The figure shows three views and two pictorial views of one solid part (mm, origin at its lowest corner). Answer the questions. Coordinates: 2 decimals unless noted, no trailing zeros. Order: outer loops, then holes, each group sorted by start corner. A loop starts at its lowest first (then second) coordinate and runs counter-clockwise, first axis right, second up. Notation, with made-up numbers: (73.25, -9.5) - (96.25, -9.5) arc R18 ccw to (96.25, 19.5) - close; hole circle Ø7 at (-17.5, 43.25). An arc over 180 degrees is marked (long way). Use one line per item in the form item = value. Start each with the question number.
Item 1: Section D-D, the plane y = 0.6 is taken. Count the separate pieces of the cut face and the enclosed holes in it, and give its area (3 significant figures).
Item 2: Section A-A, the plane z = 70 is taken. Write down the section's boundary in (x, y).
Item 3: Each of these flat-tipped pins is pushed along its axis until it touches: pin 1 Ø1.5 at (y, z) = (1, 108) entering from +X (1 decimal); pin 2 Ø5.5 at (x, z) = (11, 70) entering from +Y; pin 3 Ø2 at (y, z) = (2.5, 91.5) entering from +X; pin 4 Ø1.5 at (y, z) = (1.5, 37) entering from -X. Where does it stop, or does it pass through?
Item 4: Section B-B, the plane z = 11 is taken. Write down the section's boundary in (x, y), and give its area (3 significant figures).
Item 5: Consider line 1 along X through (y, z) = (1.85, 70); line 2 along Z through (x, y) = (109, 2.3); line 3 along Z through (x, y) = (28, 1.7). Determine where each line is inside the solid, lowest interval first. Write a range as [from, to].
Item 6: Section C-C, the plane x = 129 is taken. Write down the section's boundary in (y, z), and give its area (3 significant figures).
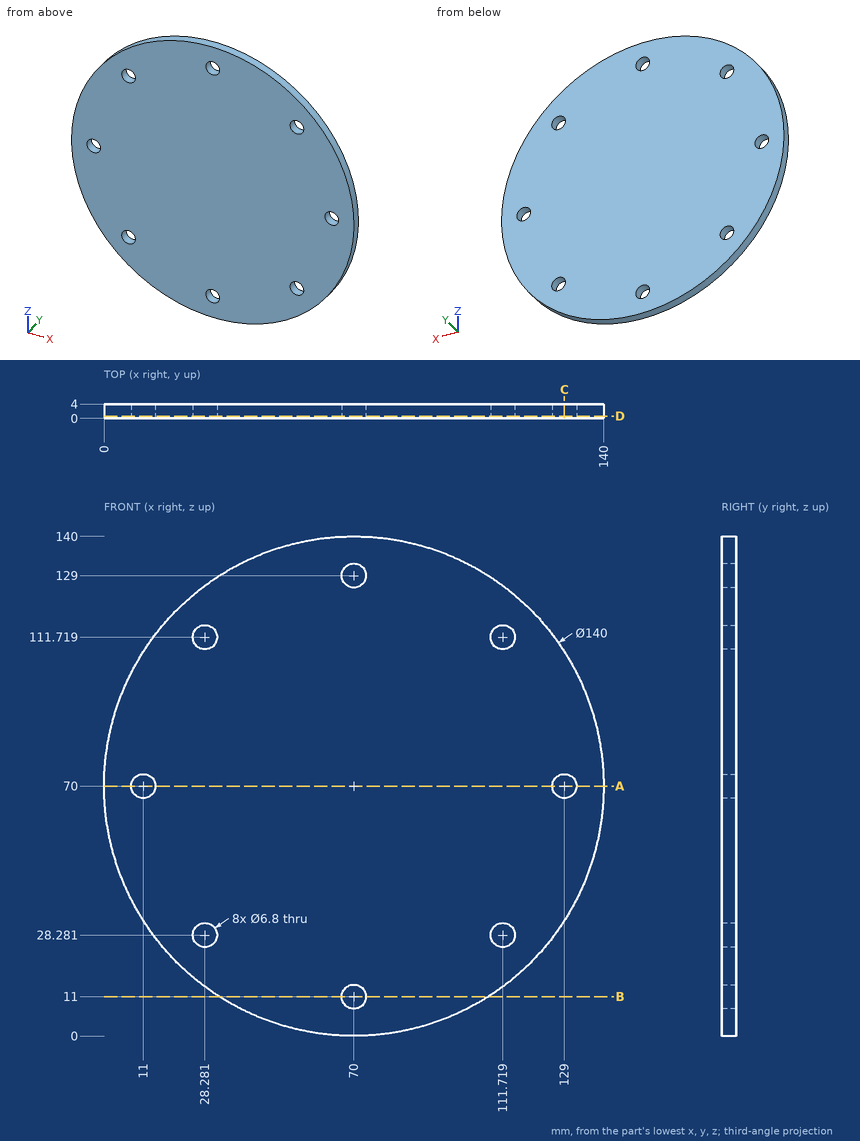
Response:
q1.separate_pieces = 1
q1.enclosed_holes = 8
q1.area = 15,100 mm2
q2.outline = (0, 0) - (7.6, 0) - (7.6, 4) - (0, 4) - close; (14.4, 0) - (125.6, 0) - (125.6, 4) - (14.4, 4) - close; (132.4, 0) - (140, 0) - (140, 4) - (132.4, 4) - close
q3.pin_1 = 129.3
q3.pin_2 = through
q3.pin_3 = 136.93
q3.pin_4 = 7.87
q4.outline = (32.33, 0) - (66.6, 0) - (66.6, 4) - (32.33, 4) - close; (73.4, 0) - (107.67, 0) - (107.67, 4) - (73.4, 4) - close
q4.area = 274 mm2
q5.line_1 = [0, 7.6], [14.4, 125.6], [132.4, 140]
q5.line_2 = [11.87, 26.24], [30.32, 109.68], [113.76, 128.13]
q5.line_3 = [14, 24.89], [31.67, 108.33], [115.11, 126]
q6.outline = (0, 32.33) - (4, 32.33) - (4, 66.6) - (0, 66.6) - close; (0, 73.4) - (4, 73.4) - (4, 107.67) - (0, 107.67) - close
q6.area = 274 mm2
